The listing builds one solid part. Answer for the finished solid, in the listing's coordinates (mm). A direction names the side the tool comes from. Give positions to 0.01 mm unless a question says otherwise; leave off trailing zeros. Write each loop counter-clockwise with the first axis right and the second up, starting at its lowest first coordinate (ties: lowest second). Pieces come first, ordered by that corner, then holes. Notation, with made-up numbers: M -36.5,58 L 5.5,58 A17 ccw 5.5,62 Z; hole C -35.75,41 d9. An arc over 180 degrees is marked long. Return JSON: item names as keys, results as strings.
from build123d import *

# Parameters (mm, degrees)
BOSS_EXTRUDE1_DEPTH = 6
FILLET1_R           = 10
SKETCH3_R           = 2.5
SKETCH3_R_2         = 4.5
SKETCH3_R_3         = 2
CUT_EXTRUDE1_DEPTH  = 87.534675131


with BuildPart() as part:
    # Sketch1 → Boss-Extrude1 (new body)
    with BuildSketch(Plane(origin=(0, 0, 0), x_dir=(1, 0, 0), z_dir=(0, 1, 0))):
        with BuildLine():
            Line((0, 0), (0, 10))
            Line((0, 10), (-30, 40))
            Line((-30, 40), (-56, 40))
            Line((-56, 40), (-56, 13.955285737))
            ThreePointArc((-56, 13.955285737), (-76.5, 0), (-56, -13.955285737))
            Line((-56, -13.955285737), (-56, -40))
            Line((-56, -40), (-30, -40))
            Line((-30, -40), (0, -10))
            Line((0, -10), (0, 0))
        make_face()
    extrude(amount=BOSS_EXTRUDE1_DEPTH)

    # Fillet1
    fillet1_edges = [part.edges().sort_by_distance(p)[0] for p in [
        (-56, 3, 13.955285737),
        (-56, 3, -13.955285737),
    ]]
    fillet(fillet1_edges, radius=FILLET1_R)

    # Sketch3 → Cut-Extrude1 (cut, through all)
    with BuildSketch(Plane(origin=(0, 6, 0), x_dir=(1, 0, 0), z_dir=(0, 1, 0))):
        with Locations(Location((-40, 0, 0), (0, 0, 270))):
            Circle(SKETCH3_R)
        with Locations(Location((-40, -30, 0), (0, 0, 270))):
            Circle(SKETCH3_R)
        with Locations(Location((-10, 0, 0), (0, 0, 270))):
            Circle(SKETCH3_R)
        with Locations(Location((-40, 30, 0), (0, 0, 270))):
            Circle(SKETCH3_R)
        with Locations(Location((-61.5, 0, 0), (0, 0, 270))):
            Circle(SKETCH3_R_2)
        with Locations(Location((-71.5, 0, 0), (0, 0, 270))):
            Circle(SKETCH3_R_3)
    extrude(amount=-CUT_EXTRUDE1_DEPTH, mode=Mode.SUBTRACT)


solid = part.part
Item 1: Determine the mould class of faces 3 (the cylindrical face through (-65.49, 3.04, 2.08)), 4 (the flat face through (-43, 3, -40)), 5 (the flat face through (-56, 3, 32)) for opening direction Z: +Z half, -Z half, draft (parallel to the pull), parting line (faces both ways), or undercut.
Geometry results:
{"face 3": "undercut", "face 4": "-Z half", "face 5": "draft"}
Item 2: A cutting plane is placed at C-C, the plane x = -10. Write down the section's boundary in (y, z), plus the area to 3 significant figures.
Geometry results:
{"outline": "M 0,-20 L 6,-20 L 6,-2.5 L 0,-2.5 Z; M 0,2.5 L 6,2.5 L 6,20 L 0,20 Z", "area": "210 mm2"}
Item 3: A cutting plane is placed at B-B, the plane y = 1.95. Write down the section's boundary in (x, z) (3 decimals), plus the area to 3 significant figures.
Geometry results:
{"outline": "M -64.2,-14.755 A10 cw -56,-24.592 L -56,-40 L -30,-40 L 0,-10 L 0,10 L -30,40 L -56,40 L -56,24.592 A10 cw -64.2,14.755 A15 ccw Z; hole C -71.5,0 d4; hole C -61.5,0 d9; hole C -40,-30 d5; hole C -40,0 d5; hole C -40,30 d5; hole C -10,0 d5", "area": "3,980 mm2"}
Item 4: Find the intervals of material crossed by line 1 (X direction, y = 4.1, z = 0); line 2 (Z direction, x = -40.5, y = 0.4); line 3 (X direction, y = 2.55, z = 30), in increasing order.
Geometry results:
{"line 1": "x = -76.5 to -73.5, -69.5 to -66, -57 to -42.5, -37.5 to -12.5, -7.5 to 0", "line 2": "z = -40 to -32.45, -27.55 to -2.45, 2.45 to 27.55, 32.45 to 40", "line 3": "x = -56 to -42.5, -37.5 to -20"}
Item 5: A cutting plane is placed at A-A, the plane x = -40. Write down the section's boundary in (y, z), plus the area to 3 significant figures.
Geometry results:
{"outline": "M 0,-40 L 6,-40 L 6,-32.5 L 0,-32.5 Z; M 0,-27.5 L 6,-27.5 L 6,-2.5 L 0,-2.5 Z; M 0,2.5 L 6,2.5 L 6,27.5 L 0,27.5 Z; M 0,32.5 L 6,32.5 L 6,40 L 0,40 Z", "area": "390 mm2"}
Item 6: Which of the six approach directions +Z, -Z, +X, -X, +Y, -Y give full straight-line access (tool end or side, diameter ignored) to faces 1 (the cylindrical face through (-76.497, 2.958, -0.292)), 2 (the flat face through (-56, 3, -32))?
Geometry results:
{"face 1": "-X, +Y, -Y", "face 2": "-Z, -X, +Y, -Y"}
Item 7: A cutting plane is placed at D-D, the plane z = 30. Write down the section's boundary in (x, y).
Geometry results:
{"outline": "M -56,0 L -42.5,0 L -42.5,6 L -56,6 Z; M -37.5,0 L -20,0 L -20,6 L -37.5,6 Z"}
Item 8: Given pin 1 Ø2 at (y, z) = (1, 3) entering from +X; pin 2 Ø2 at (y, z) = (2, 7) entering from -X; pin 3 Ø3 at (y, z) = (3, 35) entering from -X; pin 4 Ø2 at (x, y) = (-62.5, 4.5) entering from +Z, each flat-ended and moving along its own axis, determine where each tip first touches the part or whether it passes through.
Geometry results:
{"pin 1": "stops at x = 0", "pin 2": "stops at x = -75.25", "pin 3": "stops at x = -56", "pin 4": "stops at z = 15.66"}
